```python
from build123d import *

# Parameters (mm, degrees)
SKETCH2_R           = 145
SKETCH2_R_2         = 105
BOSS_EXTRUDE1_START = -50
SKETCH3_W           = 360
SKETCH3_H           = 360
SKETCH3_R           = 145
BOSS_EXTRUDE1_DEPTH = 50
FILLET1_R           = 20
SKETCH4_W           = 360
SKETCH4_H           = 360
SKETCH4_R           = 145
BOSS_EXTRUDE2_DEPTH = 50
FILLET2_R           = 20
SKETCH6_R           = 30
CUT_EXTRUDE1_DEPTH  = 10
CUT_EXTRUDE2_REACH  = 775.369
SKETCH8_R           = 15
CIRPATTERN1_COUNT   = 4
SKETCH10_R          = 30
CUT_EXTRUDE3_DEPTH  = 10
CUT_EXTRUDE4_REACH  = 890.2
SKETCH11_R          = 15
CIRPATTERN3_COUNT   = 4


with BuildPart() as part:
    # Sweep-Thin1: sweep along a path in Sketch1
    with BuildLine(Plane.XY) as sweep_thin1_path:
        Line((0, 0), (-150, 0))
        ThreePointArc((-150, 0), (-355.060966544, 84.939033456), (-440, 290))
        Line((-440, 290), (-440, 440))
    # Sketch2 → Sweep-Thin1 (sweep)
    with BuildSketch(Plane(origin=(0, 0, 0), x_dir=(0, 0, -1), z_dir=(1, 0, 0))):
        Circle(SKETCH2_R)
        Circle(SKETCH2_R_2, mode=Mode.SUBTRACT)
    sweep(path=sweep_thin1_path.line)

    # Sketch3 → Boss-Extrude1 (add)
    with BuildSketch(Plane(origin=(0, 0, 0), x_dir=(0, 0, -1), z_dir=(1, 0, 0)).offset(BOSS_EXTRUDE1_START)):
        Rectangle(SKETCH3_W, SKETCH3_H)
        with Locations(Location((0, 0, 0), (0, 0, 270))):
            Circle(SKETCH3_R, mode=Mode.SUBTRACT)
    extrude(amount=BOSS_EXTRUDE1_DEPTH)

    # Fillet1
    fillet1_edges = [part.edges().sort_by_distance(p)[0] for p in [
        (-25, -180, 180),
        (-25, 180, 180),
        (-25, 180, -180),
        (-25, -180, -180),
    ]]
    fillet(fillet1_edges, radius=FILLET1_R)

    # Sketch4 → Boss-Extrude2 (add)
    with BuildSketch(Plane(origin=(0, 440, 0), x_dir=(1, 0, 0), z_dir=(0, 1, 0))):
        with Locations((-440, 0)):
            Rectangle(SKETCH4_W, SKETCH4_H)
        with Locations(Location((-440, 0, 0), (0, 0, 180))):
            Circle(SKETCH4_R, mode=Mode.SUBTRACT)
    extrude(amount=-BOSS_EXTRUDE2_DEPTH)

    # Fillet2
    fillet2_edges = [part.edges().sort_by_distance(p)[0] for p in [
        (-620, 415, 180),
        (-620, 415, -180),
        (-260, 415, -180),
        (-260, 415, 180),
    ]]
    fillet(fillet2_edges, radius=FILLET2_R)

    # Sketch6 → Cut-Extrude1 (cut)
    with BuildSketch(Plane(origin=(0, 0, 0), x_dir=(0, 0, -1), z_dir=(1, 0, 0))):
        with Locations((-135.239614092, 130)):
            Circle(SKETCH6_R)
    cut_extrude1 = extrude(amount=-CUT_EXTRUDE1_DEPTH, mode=Mode.SUBTRACT)

    # Sketch8 → Cut-Extrude2 (cut, up to next)
    with BuildSketch(Plane(origin=(-10, 0, 0), x_dir=(0, 0, -1), z_dir=(1, 0, 0)), mode=Mode.PRIVATE) as cut_extrude2_sk1:
        with Locations((-135.239614092, 130)):
            Circle(SKETCH8_R)
    cut_extrude2_tool1 = extrude(cut_extrude2_sk1.sketch, amount=-CUT_EXTRUDE2_REACH, mode=Mode.PRIVATE) & part.part
    cut_extrude2 = cut_extrude2_tool1.solids().sort_by_distance((-10, 130, 135.239614))[0]
    add(cut_extrude2, mode=Mode.SUBTRACT)

    # CirPattern1: Cut-Extrude1, Cut-Extrude2 ×4 about axis
    cirpattern1_axis = Axis((0, 0, 0), (1, 0, 0))
    add([cut_extrude1.rotate(cirpattern1_axis, i * 360 / CIRPATTERN1_COUNT) for i in range(1, CIRPATTERN1_COUNT)], mode=Mode.SUBTRACT)
    add([cut_extrude2.rotate(cirpattern1_axis, i * 360 / CIRPATTERN1_COUNT) for i in range(1, CIRPATTERN1_COUNT)], mode=Mode.SUBTRACT)

    # Sketch10 → Cut-Extrude3 (cut)
    with BuildSketch(Plane(origin=(0, 440, 0), x_dir=(1, 0, 0), z_dir=(0, 1, 0))):
        with Locations(Location((-570, 130, 0), (0, 0, 180))):
            Circle(SKETCH10_R)
    cut_extrude3 = extrude(amount=-CUT_EXTRUDE3_DEPTH, mode=Mode.SUBTRACT)

    # Sketch11 → Cut-Extrude4 (cut, up to next)
    with BuildSketch(Plane(origin=(0, 430, 0), x_dir=(1, 0, 0), z_dir=(0, 1, 0)), mode=Mode.PRIVATE) as cut_extrude4_sk1:
        with Locations(Location((-570, 130, 0), (0, 0, 180))):
            Circle(SKETCH11_R)
    cut_extrude4_tool1 = extrude(cut_extrude4_sk1.sketch, amount=-CUT_EXTRUDE4_REACH, mode=Mode.PRIVATE) & part.part
    cut_extrude4 = cut_extrude4_tool1.solids().sort_by_distance((-570, 430, -130))[0]
    add(cut_extrude4, mode=Mode.SUBTRACT)

    # CirPattern3: Cut-Extrude3, Cut-Extrude4 ×4 about axis
    cirpattern3_axis = Axis((-440, 0, 0), (0, 1, 0))
    add([cut_extrude3.rotate(cirpattern3_axis, i * 360 / CIRPATTERN3_COUNT) for i in range(1, CIRPATTERN3_COUNT)], mode=Mode.SUBTRACT)
    add([cut_extrude4.rotate(cirpattern3_axis, i * 360 / CIRPATTERN3_COUNT) for i in range(1, CIRPATTERN3_COUNT)], mode=Mode.SUBTRACT)


solid = part.part
```
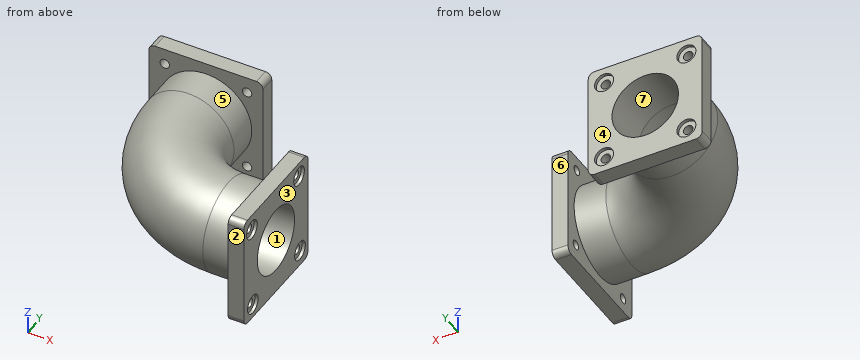
Could you check a few things on this model? Use its own coordinates, in mm. Face numbers are marked on the shaded views. A direction names the side the tool comes from. Round coordinates to 2 decimals unless told otherwise and drop trailing zeros. Loops run counter-clockwise (first coordinate to the right, second up) from the corner with the lowest first, then second, coordinate; pieces in that order, holes last. Notation, with made-up numbers: (-7.5, 41.5) -> (31.5, 41.5) arc R26 cw to (31.5, 57.5) -> close; hole circle Ø9 at (27.5, 17.25). An arc over 180 degrees is marked (long way). One line per question, with ' | ' between items.
(1) If we section it at A-A on z = 38: List the corners of the cut face in (x, y) for me, and give its area (3 significant figures).
Model answer:
outline: (-620, 390) -> (-579.93, 390) -> (-579.93, 290) arc R429.93 ccw to (-150, -139.93) -> (-50, -139.93) -> (-50, -180) -> (0, -180) -> (0, -97.88) -> (-150, -97.88) arc R387.88 cw to (-537.88, 290) -> (-537.88, 440) -> (-620, 440) -> close; (-342.12, 290) arc R192.12 ccw to (-150, 97.88) -> (0, 97.88) -> (0, 180) -> (-50, 180) -> (-50, 139.93) -> (-150, 139.93) arc R150.07 cw to (-300.07, 290) -> (-300.07, 390) -> (-260, 390) -> (-260, 440) -> (-342.12, 440) -> close | area: 71,600 mm^2
(2) For pin 1 Ø18 at (x, z) = (-570, -130) entering from -Y; pin 2 Ø1.5 at (y, z) = (-37.5, -131) entering from +X; pin 3 Ø18 at (y, z) = (-141, 136.5) entering from +X; pin 4 Ø5 at (y, z) = (235, -75) entering from -X, each with a flat end and sliding along its axis, tell me the tip position at first contact or that it passes through.
Model answer:
pin 1: passes through | pin 2: stops at x = 0 | pin 3: stops at x = -10 | pin 4: stops at x = -561.96
(3) If we section it at B-B on y = 130: Count the separate pieces of the cut face and the enclosed holes in it, and give its area (3 significant figures).
Model answer:
separate pieces: 3 | enclosed holes: 1 | area: 74,300 mm^2
(4) Thinking about a two-plate mould opening in Y: for the marked faces 1, 2 and 3, which applies, released by +Y, released by -Y, zero draft, split by the parting line, or undercut?
Model answer:
face 1: undercut | face 2: released by -Y | face 3: zero draft
(5) If I drill on probe 1 along X at (y, z) = (414.5, -130); probe 2 along Z at (x, y) = (-310, 419); probe 3 along X at (y, z) = (154, -73), over which ranges is the centre line in solid material (lowest first)?
Model answer:
probe 1: x = -620 to -585, -555 to -325, -295 to -260 | probe 2: z = -180 to -145, -115 to 115, 145 to 180 | probe 3: x = -542.38 to -489.23, -315.91 to -242.93, -50 to 0
(6) For the marked faces 4, 5, 6 and 7, which set-ups out of +Z, -Z, +X, -X, +Y, -Y let a thin tool reach every point of the face, with its end or its side?
Model answer:
face 4: +Z, -Z, +X, -X, +Y | face 5: none | face 6: +Z, -Z, +X, +Y | face 7: +Y
